from build123d import *

# Parameters (mm, degrees)
BOSS_EXTRUDE1_DEPTH = 10
SKETCH2_R           = 2
CUT_EXTRUDE1_DEPTH  = 65.807406984
FILLET1_R           = 5
SKETCH3_R           = 2
CUT_EXTRUDE2_DEPTH  = 65.807406984


with BuildPart() as part:
    # Sketch1 → Boss-Extrude1 (new body)
    with BuildSketch(Plane.XY):
        Polygon((40, 0), (50, 0), (50, 40), (0, 40), (0, 0), (10, 0), (10, 17), (40, 17), align=None)
    extrude(amount=BOSS_EXTRUDE1_DEPTH)

    # Sketch2 → Cut-Extrude1 (cut, through all)
    with BuildSketch(Plane(origin=(50, 0, 0), x_dir=(0, 0, -1), z_dir=(1, 0, 0))):
        with Locations((-5, 5)):
            Circle(SKETCH2_R)
    extrude(amount=-CUT_EXTRUDE1_DEPTH, mode=Mode.SUBTRACT)

    # Fillet1
    fillet1_edges = [part.edges().sort_by_distance(p)[0] for p in [
        (25, 17, 10),
    ]]
    fillet(fillet1_edges, radius=FILLET1_R)

    # Sketch3 → Cut-Extrude2 (cut, through all)
    with BuildSketch(Plane.ZY):
        with Locations((5, 35)):
            Circle(SKETCH3_R)
    extrude(amount=-CUT_EXTRUDE2_DEPTH, mode=Mode.SUBTRACT)


solid = part.part
Model file for the job. Use its own axes, mm. A direction names the side the tool comes from. Round coordinates to 2 decimals unless told otherwise and drop trailing zeros. Loops run counter-clockwise (first coordinate to the right, second up) from the corner with the lowest first, then second, coordinate; pieces in that order, holes last. Notation, with made-up numbers: (-35.5, -39.75) -> (14.5, -39.75) arc R15 cw to (14.5, -35.75) -> close; hole circle Ø8 at (11.25, 1.25). An arc over 180 degrees is marked (long way). Answer as CSV lines item,"result". Start each with the question number.
1) Pin check, flat tips, straight feed: P1, Ø5, axis at y = 9, z = 5, coming from the -X side; P2, Ø5.5, axis at x = 21, z = 3, coming from the -Y side. Stop position of each tip, or through.
2) Slice it at D-D (y = 5). List the corners of the cut face in (x, z), plus the area to 3 significant figures.
3) Tool access for faces 4 (the face through (25, 17, 2)), 5 (the face through (45, 0, 5)): list every direction of +Z, -Z, +X, -X, +Y, -Y with a clear straight run to the whole face (end or side of a thin tool).
4) Probe line 1 along Y through (x, z) = (6, 5); line 2 along X through (y, z) = (12, 9); line 3 along Y through (x, z) = (6.5, 4.5). List the from-to ranges inside material, lowest first.
5) Slice it at B-B (x = 13). List the corners of the cut face in (y, z).
6) Mould opens along X. For faces 1 (the face through (25, 25, 0)), 2 (the face through (50, 20, 5)), 3 (the face through (25, 19, 9)) say: +X half, -X half, draft (parallel to the pull), parting line (faces both ways), or undercut.
7) Slice it at A-A (y = 35). List the corners of the cut face in (x, z).
8) Slice it at C-C (z = 4). List the corners of the cut face in (x, y), plus the area to 3 significant figures.
Filled in:
1,P1,"stops at x = 0"
1,P2,"stops at y = 17"
2,outline,"(0, 0) -> (10, 0) -> (10, 3) -> (0, 3) -> close; (0, 7) -> (10, 7) -> (10, 10) -> (0, 10) -> close; (40, 0) -> (50, 0) -> (50, 3) -> (40, 3) -> close; (40, 7) -> (50, 7) -> (50, 10) -> (40, 10) -> close"
2,area,"120 mm2"
3,face 4,"+Z, -Z, -Y"
3,face 5,"+Z, -Z, +X, -X, -Y"
4,line 1,"y = 0 to 3, 7 to 33, 37 to 40"
4,line 2,"x = 0 to 10, 40 to 50"
4,line 3,"y = 0 to 3.06, 6.94 to 33.06, 36.94 to 40"
5,outline,"(17, 0) -> (40, 0) -> (40, 10) -> (22, 10) arc R5 ccw to (17, 5) -> close; hole circle Ø4 at (35, 5)"
6,face 1,"draft"
6,face 2,"+X half"
6,face 3,"undercut"
7,outline,"(0, 0) -> (50, 0) -> (50, 3) -> (0, 3) -> close; (0, 7) -> (50, 7) -> (50, 10) -> (0, 10) -> close"
8,outline,"(0, 0) -> (10, 0) -> (10, 3.27) -> (0, 3.27) -> close; (0, 6.73) -> (10, 6.73) -> (10, 17) -> (40, 17) -> (40, 6.73) -> (50, 6.73) -> (50, 33.27) -> (0, 33.27) -> close; (0, 36.73) -> (50, 36.73) -> (50, 40) -> (0, 40) -> close; (40, 0) -> (50, 0) -> (50, 3.27) -> (40, 3.27) -> close"
8,area,"1,250 mm2"
